from build123d import *

# Parameters (mm, degrees)
SKETCH1_W           = 210
SKETCH1_H           = 105
BOSS_EXTRUDE1_DEPTH = 6
SKETCH2_W           = 210
SKETCH2_H           = 6
BOSS_EXTRUDE2_DEPTH = 126
SKETCH3_W           = 111
SKETCH3_H           = 126
BOSS_EXTRUDE3_DEPTH = 6
CUT_EXTRUDE2_DEPTH  = 6
SKETCH7_R           = 9
CUT_EXTRUDE3_DEPTH  = 24
SKETCH8_W           = 72.8
SKETCH8_H           = 73.25
CUT_EXTRUDE4_DEPTH  = 24
SKETCH9_W           = 80
SKETCH9_H           = 33
CUT_EXTRUDE5_DEPTH  = 24
FILLET1_R           = 20
SKETCH11_W          = 80
SKETCH11_H          = 33
SKETCH11_W_2        = 76
SKETCH11_H_2        = 29
BOSS_EXTRUDE4_DEPTH = 2
FILLET2_R           = 2
SKETCH12_R          = 1.5
CUT_EXTRUDE6_DEPTH  = 20
SKETCH13_R          = 1.5
CUT_EXTRUDE7_DEPTH  = 25


with BuildPart() as part:
    # Sketch1 → Boss-Extrude1 (new body)
    with BuildSketch(Plane(origin=(0, 0, 0), x_dir=(1, 0, 0), z_dir=(0, 1, 0))):
        with Locations((105, 52.5)):
            Rectangle(SKETCH1_W, SKETCH1_H)
    extrude(amount=BOSS_EXTRUDE1_DEPTH)

    # Sketch2 → Boss-Extrude2 (add)
    with BuildSketch(Plane.XZ):
        with Locations((105, -108)):
            Rectangle(SKETCH2_W, SKETCH2_H)
    extrude(amount=-BOSS_EXTRUDE2_DEPTH)

    # Sketch3 → Boss-Extrude3 (add)
    with BuildSketch(Plane(origin=(210, 0, 0), x_dir=(0, 0, -1), z_dir=(1, 0, 0))):
        with Locations((55.5, 63)):
            Rectangle(SKETCH3_W, SKETCH3_H)
    extrude(amount=BOSS_EXTRUDE3_DEPTH)

    # Sketch6 → Cut-Extrude2 (cut)
    with BuildSketch(Plane(origin=(216, 0, 0), x_dir=(0, 0, -1), z_dir=(1, 0, 0))):
        Polygon((0, 58.7), (47.2, 126), (0, 126), align=None)
    extrude(amount=-CUT_EXTRUDE2_DEPTH, mode=Mode.SUBTRACT)

    # Sketch7 → Cut-Extrude3 (cut)
    with BuildSketch(Plane(origin=(0, 6, 0), x_dir=(1, 0, 0), z_dir=(0, 1, 0))):
        with Locations(Location((157.5, 30, 0), (0, 0, 270))):
            Circle(SKETCH7_R)
    extrude(amount=-CUT_EXTRUDE3_DEPTH, mode=Mode.SUBTRACT)

    # Sketch8 → Cut-Extrude4 (cut)
    with BuildSketch(Plane(origin=(216, 0, 0), x_dir=(0, 0, -1), z_dir=(1, 0, 0))):
        with Locations((68.6, 50)):
            Rectangle(SKETCH8_W, SKETCH8_H)
    extrude(amount=-CUT_EXTRUDE4_DEPTH, mode=Mode.SUBTRACT)

    # Sketch9 → Cut-Extrude5 (cut)
    with BuildSketch(Plane(origin=(0, 6, 0), x_dir=(1, 0, 0), z_dir=(0, 1, 0))):
        with Locations((85, 46)):
            Rectangle(SKETCH9_W, SKETCH9_H)
    extrude(amount=-CUT_EXTRUDE5_DEPTH, mode=Mode.SUBTRACT)

    # Fillet1
    fillet1_edges = [part.edges().sort_by_distance(p)[0] for p in [
        (213, 58.7, 0),
    ]]
    fillet(fillet1_edges, radius=FILLET1_R)

    # Sketch11 → Boss-Extrude4 (add)
    with BuildSketch(Plane.XZ):
        with Locations((85, -46)):
            Rectangle(SKETCH11_W, SKETCH11_H)
        with Locations((85, -46)):
            Rectangle(SKETCH11_W_2, SKETCH11_H_2, mode=Mode.SUBTRACT)
    extrude(amount=-BOSS_EXTRUDE4_DEPTH)

    # Fillet2
    fillet2_edges = [part.edges().sort_by_distance(p)[0] for p in [
        (85, 2, -31.5),
        (123, 2, -46),
        (85, 2, -60.5),
        (47, 2, -46),
    ]]
    fillet(fillet2_edges, radius=FILLET2_R - 0.0001)  # a hair under: the kernel refuses the full size

    # Sketch12 → Cut-Extrude6 (cut)
    with BuildSketch(Plane.XY):
        with Locations((201, 3)):
            Circle(SKETCH12_R)
        with Locations((186, 3)):
            Circle(SKETCH12_R)
    extrude(amount=-CUT_EXTRUDE6_DEPTH, mode=Mode.SUBTRACT)

    # Sketch13 → Cut-Extrude7 (cut)
    with BuildSketch(Plane(origin=(0, 126, 0), x_dir=(1, 0, 0), z_dir=(0, 1, 0))):
        with Locations(Location((15, 108, 0), (0, 0, 270))):
            Circle(SKETCH13_R)
        with Locations(Location((30, 108, 0), (0, 0, 270))):
            Circle(SKETCH13_R)
    extrude(amount=-CUT_EXTRUDE7_DEPTH, mode=Mode.SUBTRACT)


solid = part.part
Input: part model. Units: mm. Frame: model coordinates. A direction names the side the tool comes from. Round coordinates to 2 decimals unless told otherwise and drop trailing zeros. Write each loop counter-clockwise with the first axis right and the second up, starting at its lowest first coordinate (ties: lowest second). Pieces come first, ordered by that corner, then holes.
1) Contact query for flat-ended pins moving along their axis: P1, Ø6, axis at x = 103, y = 82.5, coming from the +Z side; P2, Ø1.5, axis at x = 163, z = -97, coming from the +Y side; P3, Ø14.5, axis at x = 157.5, z = -30, coming from the +Y side. Output: stop coordinate, or through.
2) Reachability of faces 5 (the flat face through (210, 80, -28)), 6 (the flat face through (213, 13.375, -68)), 7 (the flat face through (0, 44, -109)) from +Z, -Z, +X, -X, +Y, -Y: full face, straight path, thin tool, end or side. Return the list, or none.
3) Cut plane D-D (x = 137.5). Return the cut outline in (y, z), then the cut area to 3 significant figures.
4) Cut plane A-A (y = 16.5). Return the cut outline in (x, z), then the cut area to 3 significant figures.
5) Cut plane C-C (y = 118.5). Return the cut outline in (x, z), then the cut area to 3 significant figures.
6) Ray query, L1, parallel to X at y = 3.5, z = -30; L2, parallel to Y at x = 201, z = -15.5; L3, parallel to Y at x = 126.5, z = -40. Return the intervals inside material, ascending.
7) Draft query along Z for faces 1 (the flat face through (106, 62, -111)), 2 (the flat face through (104, 6, -65)), 3 (the flat face through (213, 86.625, -68)), 4 (the cylindrical face through (212.958, 58.325, -0.902)). Return one class per face: pulls with the +Z half, pulls with the -Z half, needs draft (parallel to the pull), parting line crosses it, or undercut.
Geometry says:
1. P1: stops at z = -105
1. P2: stops at y = 6
1. P3: passes through
2. face 5: +Z, -X, +Y
2. face 6: +X, -X
2. face 7: +Z, -Z, -X, +Y, -Y
3. outline: (0, -111) - (126, -111) - (126, -105) - (6, -105) - (6, 0) - (0, 0) - close
3. area: 1,390 mm2
4. outline: (0, -111) - (216, -111) - (216, -105) - (0, -105) - close; (210, -32.2) - (216, -32.2) - (216, 0) - (210, 0) - close
4. area: 1,490 mm2
5. outline: (0, -111) - (216, -111) - (216, -41.94) - (210, -41.94) - (210, -105) - (0, -105) - close; hole circle Ø3 at (15, -108); hole circle Ø3 at (30, -108)
5. area: 1,660 mm2
6. L1: x = 0 to 45, 125 to 148.5, 166.5 to 216
6. L2: y = 0 to 1.5, 4.5 to 6
6. L3: y = 0 to 6
7. face 1: pulls with the -Z half
7. face 2: needs draft
7. face 3: undercut
7. face 4: pulls with the +Z half
